Read the model definition and answer for the solid it produces. Units are mm, in the model's axes. Round coordinates to 2 decimals unless told otherwise and drop trailing zeros. Write each loop counter-clockwise with the first axis right and the second up, starting at its lowest first coordinate (ties: lowest second). Pieces come first, ordered by that corner, then holes. Notation, with made-up numbers: (37, -31.75) - (59, -31.75) arc R8 ccw to (59, -21.75) - close; hole circle Ø11 at (-14.75, 64). An arc over 180 degrees is marked (long way). Answer as CSV lines item,"result". Start each with the question number.
1) Consider line 1 along X through (y, z) = (1.8, 13); line 2 along X through (y, z) = (1.1, -17); line 3 along X through (y, z) = (1.95, -17.5). Determine where each line is inside the solid, lowest interval first.
2) For a pull along Z with two mould halves and no side action, classify faces 1 (the flat face through (-35.282, 1, 4)), 2 (the cylindrical face through (43.39, 1.52, -16.19)), 3 (the cylindrical face through (25.983, 1.521, 13.922)), 4 (the cylindrical face through (84.12, 1.52, -21.31)) as +Z half, -Z half, draft (parallel to the pull), parting line (faces both ways), or undercut.
3) Find section A-A on z = -16.5. Determine the outline of the cut face in (x, y).
4) This flat-tipped pin is pushed along its axis until it touches: pin 1 (2.5 mm diameter, centred on x = 44.72, z = -16.88, fed in from +Y). Where does it stop, or does it pass through?
from build123d import *

# Parameters (mm, degrees)
SKETCH_1_W          = 120
SKETCH_1_H          = 49
EXTRUDE_1_DEPTH     = 3
SKETCH_2_R          = 1.5
CUT_EXTRUDE_1_DEPTH = 3
FILLET_1_R          = 2


with BuildPart() as part:
    # 草图1 → 凸台-拉伸1 (new body)
    with BuildSketch(Plane(origin=(0, 0, 0), x_dir=(1, 0, 0), z_dir=(0, 1, 0))):
        with Locations((24.718351515, -2.615392567)):
            Rectangle(SKETCH_1_W, SKETCH_1_H)
    extrude(amount=EXTRUDE_1_DEPTH)

    # 草图2 → 切除-拉伸1 (cut)
    with BuildSketch(Plane(origin=(0, 3, 0), x_dir=(1, 0, 0), z_dir=(0, 1, 0))):
        with Locations(Location((4.718351515, 16.884607433, 0), (0, 0, 270))):
            Circle(SKETCH_2_R)
        with Locations(Location((44.718351515, 16.884607433, 0), (0, 0, 270))):
            Circle(SKETCH_2_R)
        with Locations(Location((24.718351515, -13.115392567, 0), (0, 0, 270))):
            Circle(SKETCH_2_R)
    extrude(amount=-CUT_EXTRUDE_1_DEPTH, mode=Mode.SUBTRACT)

    # 圆角1
    fillet_1_edges = [part.edges().sort_by_distance(p)[0] for p in [
        (-35.281648485, 1.5, -21.884607433),
        (84.718351515, 1.5, -21.884607433),
    ]]
    fillet(fillet_1_edges, radius=FILLET_1_R)


solid = part.part
Check values:
1,line 1,"x = -35.28 to 23.22, 26.21 to 84.72"
1,line 2,"x = -35.28 to 3.22, 6.21 to 43.22, 46.21 to 84.72"
1,line 3,"x = -35.28 to 3.35, 6.09 to 43.35, 46.09 to 84.72"
2,face 1,"draft"
2,face 2,"undercut"
2,face 3,"undercut"
2,face 4,"-Z half"
3,outline,"(-35.28, 0) - (3.27, 0) - (3.27, 3) - (-35.28, 3) - close; (6.17, 0) - (43.27, 0) - (43.27, 3) - (6.17, 3) - close; (46.17, 0) - (84.72, 0) - (84.72, 3) - (46.17, 3) - close"
4,pin 1,"passes through"
